Geometry: final body of the model. Coordinates: model frame, mm. A direction names the side the tool comes from. Coordinates: 2 decimals unless noted, no trailing zeros. Loops run counter-clockwise (first coordinate to the right, second up) from the corner with the lowest first, then second, coordinate; pieces in that order, holes last. Notation, with made-up numbers: (38.25, -35) - (59.25, -35) arc R28 cw to (59.25, 0) - close; hole circle Ø2 at (69, 45.25). An arc over 180 degrees is marked (long way). Put each result on its own line as item: value. Start each with the question number.
1) Section C-C on x = 4.25. Output: boundary loops of the cut face in (y, z).
2) Section B-B on y = -3. Output: boundary loops of the cut face in (x, z).
3) Draft query along Y for faces 1 (the flat face through (0, -3, 5.461)), 2 (the flat face through (0.034, -11.611, 14.484)), 3 (the flat face through (0.034, 12.46, 14.923)), 4 (the cylindrical face through (-0.322, 2.455, 14.484)). Return one class per face: +Y half, -Y half, draft (parallel to the pull), parting line (faces both ways), or undercut.
4) Section D-D on z = 3.5. Output: boundary loops of the cut face in (x, y).
5) Reachability of faces 5 (the flat face through (-2.413, 8.8, 15.1)), 6 (the cylindrical face through (-0.322, 2.455, 5.736)), 7 (the flat face through (10.749, 6.245, 14.948)), 8 (the flat face through (2.413, -8.6, 15.1)), 9 (the flat face through (8.696, 2.234, 15.145)) from +Z, -Z, +X, -X, +Y, -Y: full face, straight path, thin tool, end or side. Return the list, or none.
6) Contact query for flat-ended pins moving along their axis: pin 1 Ø8 at (y, z) = (-7, 10.5) entering from -X; pin 2 Ø8 at (y, z) = (-2, 20.5) entering from -X; pin 3 Ø2 at (y, z) = (-10.5, 14.5) entering from +X; pin 4 Ø0.5 at (y, z) = (9.5, 14.5) entering from +X. Output: stop coordinate, or through.
7) Section A-A on x = 0. Output: boundary loops of the cut face in (y, z), and give its area (3 significant figures).
8) Material intervals for line 1 along Z through (x, y) = (1.75, 6.5); line 2 along Z through (x, y) = (3.75, -8.5); line 3 along Z through (x, y) = (-9.5, -6), sorted ascending. Write a range as from..to.
```python
from build123d import *

# Parameters (mm, degrees)
SKETCH1_R           = 13.462
BOSS_EXTRUDE1_DEPTH = 5.461
SKETCH2_R           = 2.4765
BOSS_EXTRUDE2_DEPTH = 26.3144
SKETCH3_R           = 13.462
BOSS_EXTRUDE3_DEPTH = 8.0264
BOSS_EXTRUDE4_DEPTH = 2.413
CIRPATTERN1_COUNT   = 3
SKETCH5_R           = 15.79013095
SKETCH5_R_2         = 13.462
CUT_EXTRUDE1_DEPTH  = 0.190772


with BuildPart() as part:
    # Sketch1 → Boss-Extrude1 (new body)
    with BuildSketch(Plane.XY):
        Circle(SKETCH1_R)
    extrude(amount=BOSS_EXTRUDE1_DEPTH)

    # Sketch2 → Boss-Extrude2 (add)
    with BuildSketch(Plane.XY.offset(5.461)):
        Circle(SKETCH2_R)
    extrude(amount=BOSS_EXTRUDE2_DEPTH)

    # Sketch3 → Boss-Extrude3 (add)
    with BuildSketch(Plane.XY.offset(6.0198)):
        Circle(SKETCH3_R)
    extrude(amount=BOSS_EXTRUDE3_DEPTH)

    # Sketch4 → Boss-Extrude4 (add, symmetric)
    with BuildSketch(Plane(origin=(0, 0, 0), x_dir=(0, 0, -1), z_dir=(1, 0, 0))):
        Polygon((-14.0462, 13.462), (-15.8242, 11.43), (-15.8242, -11.43), (-14.0462, -13.462), (-14.0462, -12.111971482), (-14.9352, -11.095971482), (-14.9352, 11.095971482), (-14.0462, 12.111971482), align=None)
    boss_extrude4 = extrude(amount=BOSS_EXTRUDE4_DEPTH, both=True)

    # CirPattern1: Boss-Extrude4 ×3 about axis
    cirpattern1_axis = Axis((0, 0, 0), (0, 0, 1))
    for i in range(1, CIRPATTERN1_COUNT):
        add(boss_extrude4.rotate(cirpattern1_axis, i * 360 / CIRPATTERN1_COUNT))

    # Sketch5 → Cut-Extrude1 (cut)
    with BuildSketch(Plane.XY.offset(14.0462)):
        Circle(SKETCH5_R)
        Circle(SKETCH5_R_2, mode=Mode.SUBTRACT)
    extrude(amount=CUT_EXTRUDE1_DEPTH, mode=Mode.SUBTRACT)


solid = part.part
```
Answer block:
1. outline: (-12.77, 0) - (12.77, 0) - (12.77, 5.46) - (-12.77, 5.46) - close; (-12.77, 6.02) - (12.77, 6.02) - (12.77, 14.05) - (-12.77, 14.05) - close; (-5.24, 14.94) - (5.24, 14.94) - (5.24, 15.82) - (-5.24, 15.82) - close
2. outline: (-13.12, 0) - (13.12, 0) - (13.12, 5.46) - (-13.12, 5.46) - close; (-13.12, 6.02) - (13.12, 6.02) - (13.12, 14.05) - (-13.12, 14.05) - close; (-10.02, 14.94) - (10.02, 14.94) - (10.02, 15.82) - (-10.02, 15.82) - close
3. face 1: draft
3. face 2: undercut
3. face 3: +Y half
3. face 4: undercut
4. outline: circle Ø26.92 at (0, 0)
5. face 5: +Z, +Y
5. face 6: none
5. face 7: +Z, +X, +Y
5. face 8: +Z, -Y
5. face 9: +Z, +X
6. pin 1: stops at x = -13.12
6. pin 2: stops at x = -2.48
6. pin 3: stops at x = 9.43
6. pin 4: passes through
7. outline: (-13.46, 0) - (13.46, 0) - (13.46, 5.46) - (2.48, 5.46) - (2.48, 6.02) - (13.46, 6.02) - (13.46, 14.05) - (11.43, 15.82) - (2.48, 15.82) - (2.48, 31.78) - (-2.48, 31.78) - (-2.48, 15.82) - (-11.43, 15.82) - (-13.46, 14.05) - (-13.46, 6.02) - (-2.48, 6.02) - (-2.48, 5.46) - (-13.46, 5.46) - close; hole (-12.11, 14.05) - (-2.48, 14.05) - (-2.48, 14.94) - (-11.1, 14.94) - close; hole (2.48, 14.05) - (12.11, 14.05) - (11.1, 14.94) - (2.48, 14.94) - close
7. area: 473 mm²
8. line 1: z = 0..5.46, 6.02..14.05, 14.94..15.82
8. line 2: z = 0..5.46, 6.02..14.05
8. line 3: z = 0..5.46, 6.02..14.05, 14.82..15.82
